Solid Edge part; units mm, degrees
sketch "Sketch1" plane through (0, 0, 0) normal (0, 0, 1) x (1, 0, 0)
  line L0 (0, 0) -> (73, 0)
  line L1 (73, 0) -> (73, 73)
  line L2 (73, 73) -> (0, 73)
  line L3 (0, 73) -> (0, 0)
extrude "Protrusion1" add sketch "Sketch1" along normal blind 23
sketch "Sketch2" plane through (36.5, 36.5, 23) normal (0, 0, 1) x (1, 0, 0)
  circle A0 centre (32.5, 32.5) radius 1.65
  circle A1 centre (32.5, -32.5) radius 1.65
  circle A2 centre (-32.5, -32.5) radius 1.65
  circle A3 centre (-32.5, 32.5) radius 1.65
extrude "ExtrudedCutout_1" cut sketch "Sketch2" against normal blind 23
sketch "Sketch3" plane through (36.5, 36.5, 23) normal (0, 0, 1) x (1, 0, 0)
  circle A0 centre (32.5, 32.5) radius 5.6569
  circle A1 centre (-32.5, -32.5) radius 5.6569
  circle A2 centre (32.5, -32.5) radius 5.6569
  circle A3 centre (-32.5, 32.5) radius 5.6569
extrude "ExtrudedCutout_2" cut sketch "Sketch3" against normal blind 21.5
CAD build for the part. Positions are in the model's coordinates, mm. A direction names the side the tool comes from. Give positions to 0.01 mm unless a question says otherwise; leave off trailing zeros. Loops run counter-clockwise (first coordinate to the right, second up) from the corner with the lowest first, then second, coordinate; pieces in that order, holes last. Notation, with made-up numbers: (-32.75, 7) - (-0.75, 7) arc R4 ccw to (-0.75, 12) - close; hole circle Ø1 at (-15.5, -0.5). An arc over 180 degrees is marked (long way). Put each result on its own line as item: value.
Q1. Slice it at A-A (y = 4). Give the cut face in (x, z).
Filled in:
outline: (0, 0) - (2.35, 0) - (2.35, 1.5) - (0, 1.5) - close; (5.65, 0) - (67.35, 0) - (67.35, 1.5) - (63.34, 1.5) - (63.34, 23) - (9.66, 23) - (9.66, 1.5) - (5.65, 1.5) - close; (70.65, 0) - (73, 0) - (73, 1.5) - (70.65, 1.5) - close
Q2. Slice it at D-D (z = 15). Give the cut face in (x, y), plus the area to 3 significant figures.
Filled in:
outline: (0, 8) arc R5.66 cw to (8, 0) - (65, 0) arc R5.66 cw to (73, 8) - (73, 65) arc R5.66 cw to (65, 73) - (8, 73) arc R5.66 cw to (0, 65) - close
area: 5,000 mm²
Q3. Slice it at C-C (y = 66). Give the cut face in (x, z).
Filled in:
outline: (0, 0) - (73, 0) - (73, 1.5) - (64.2, 1.5) - (64.2, 23) - (8.8, 23) - (8.8, 1.5) - (0, 1.5) - close
Q4. Probe line 1 along Y through (x, z) = (69, 0.7); line 2 along X through (y, z) = (5.5, 2.5). List the from-to ranges inside material, lowest first.
Filled in:
line 1: y = 0 to 2.35, 5.65 to 67.35, 70.65 to 73
line 2: x = 9.45 to 63.55
Q5. Tool access for faces 5 (the face through (68.6, 67.4, 0.8)), 6 (the face through (65, 65, 12)): list every direction of +Z, -Z, +X, -X, +Y, -Y with a clear straight run to the whole face (end or side of a thin tool).
Filled in:
face 5: +Z, -Z
face 6: +Z
Q6. Flat gauge pins, fed straight in: pin 1 (6 mm diameter, centred on x = 52, y = 56, fed in from -Z); pin 2 (5.5 mm diameter, centred on x = 69, y = 69, fed in from +Z); pin 3 (2.5 mm diameter, centred on x = 4, y = 4, fed in from -Z). Where does each tip first touch, or does it go through?
Filled in:
pin 1: stops at z = 0
pin 2: stops at z = 1.5
pin 3: passes through
Q7. Mould opens along Y. For faces 1 (the face through (3.6, 67.4, 0.8)), 2 (the face through (36, 0, 11)), 3 (the face through (36, 37, 0)), 4 (the face through (8, 8, 12)) say: pulls with the +Y half, pulls with the -Y half, needs draft (parallel to the pull), parting line crosses it, or undercut.
Filled in:
face 1: undercut
face 2: pulls with the -Y half
face 3: needs draft
face 4: undercut
